from build123d import *

# Parameters (mm, degrees)
SKETCH_1_W      = 126
SKETCH_1_H      = 37
SKETCH_1_R      = 1.5
SKETCH_1_R_2    = 2.5
EXTRUDE_1_DEPTH = 6


with BuildPart() as part:
    # 草图1 → 凸台-拉伸1 (new body)
    with BuildSketch(Plane.XY):
        Rectangle(SKETCH_1_W, SKETCH_1_H)
        with Locations((-57, 12.5)):
            Circle(SKETCH_1_R, mode=Mode.SUBTRACT)
        with Locations((-33, 12.5)):
            Circle(SKETCH_1_R, mode=Mode.SUBTRACT)
        with Locations((-57, -12.5)):
            Circle(SKETCH_1_R, mode=Mode.SUBTRACT)
        with Locations((-33, -12.5)):
            Circle(SKETCH_1_R, mode=Mode.SUBTRACT)
        with Locations((33, 12.5)):
            Circle(SKETCH_1_R, mode=Mode.SUBTRACT)
        with Locations((57, 12.5)):
            Circle(SKETCH_1_R, mode=Mode.SUBTRACT)
        with Locations((57, -12.5)):
            Circle(SKETCH_1_R, mode=Mode.SUBTRACT)
        with Locations((33, -12.5)):
            Circle(SKETCH_1_R, mode=Mode.SUBTRACT)
        with Locations((-5.656854249, 5.656854249)):
            Circle(SKETCH_1_R, mode=Mode.SUBTRACT)
        with Locations((5.656854249, 5.656854249)):
            Circle(SKETCH_1_R, mode=Mode.SUBTRACT)
        with Locations((-5.656854249, -5.656854249)):
            Circle(SKETCH_1_R, mode=Mode.SUBTRACT)
        with Locations((5.656854249, -5.656854249)):
            Circle(SKETCH_1_R, mode=Mode.SUBTRACT)
        Circle(SKETCH_1_R_2, mode=Mode.SUBTRACT)
    extrude(amount=EXTRUDE_1_DEPTH)


solid = part.part
Geometry: final body of the model. Coordinates: model frame, mm. Round coordinates to 2 decimals unless told otherwise and drop trailing zeros. Order: outer loops, then holes, each group sorted by start corner. A loop starts at its lowest first (then second) coordinate and runs counter-clockwise, first axis right, second up. Notation, with made-up numbers: (-9.5, 37.25) -> (-1.5, 37.25) arc R14 ccw to (-1.5, 51.25) -> close; hole circle Ø4 at (8, -15). An arc over 180 degrees is marked (long way). Put each result on its own line as item: value. Start each with the question number.
Q1. Section C-C on x = -33. Return the cut outline in (y, z).
Q2. First-contact query: pin 1 (2.5 mm diameter, centred on x = -33, y = -12.5, fed in from +Z). Flat tip, straight axial feed; report the tip coordinate or a pass-through.
Q3. Line query: probe 1 along Y at (x, z) = (-33, 4.2); probe 2 along X at (y, z) = (4.5, 1.9); probe 3 along Y at (x, z) = (0, 2.35). Output: solid intervals per line, ascending.
Q4. Section B-B on x = 0. Return the cut outline in (y, z), and give its area (3 significant figures).
Q5. Pull-direction query (X, two-part tool) for faces 1 (the flat face through (-63, 0, 3)), 2 (the cylindrical face through (6.3, 4.3, 3)), 3 (the cylindrical face through (31.5, -12.43, 2.96)), 4 (the flat face through (63, 0, 3)); classes: +X half, -X half, draft (parallel to the pull), parting line (faces both ways), or undercut.
Q6. Section D-D on z = 1.55. Give the number of separate pieces and of enclosed holes in the cut face, and give its area (3 significant figures).
Q7. Section A-A on y = 0. Return the cut outline in (x, z), and give its area (3 significant figures).
Ans:
1. outline: (-18.5, 0) -> (-14, 0) -> (-14, 6) -> (-18.5, 6) -> close; (-11, 0) -> (11, 0) -> (11, 6) -> (-11, 6) -> close; (14, 0) -> (18.5, 0) -> (18.5, 6) -> (14, 6) -> close
2. pin 1: passes through
3. probe 1: y = -18.5 to -14, -11 to 11, 14 to 18.5
3. probe 2: x = -63 to -6.61, -4.7 to 4.7, 6.61 to 63
3. probe 3: y = -18.5 to -2.5, 2.5 to 18.5
4. outline: (-18.5, 0) -> (-2.5, 0) -> (-2.5, 6) -> (-18.5, 6) -> close; (2.5, 0) -> (18.5, 0) -> (18.5, 6) -> (2.5, 6) -> close
4. area: 192 mm2
5. face 1: -X half
5. face 2: undercut
5. face 3: undercut
5. face 4: +X half
6. separate pieces: 1
6. enclosed holes: 13
6. area: 4,560 mm2
7. outline: (-63, 0) -> (-2.5, 0) -> (-2.5, 6) -> (-63, 6) -> close; (2.5, 0) -> (63, 0) -> (63, 6) -> (2.5, 6) -> close
7. area: 726 mm2
